Autodesk Inventor part; units mm, degrees
ref_plane "YZ Plane" through (0, 0, 0) normal (1, 0, 0) x (0, 1, 0)
ref_plane "XZ Plane" through (0, 0, 0) normal (0, 1, 0) x (-1, 0, 0)
ref_plane "XY Plane" through (0, 0, 0) normal (0, 0, 1) x (1, 0, 0)
sketch "Sketch1" plane through (0, 0, 0) normal (0, 1, 0) x (-1, 0, 0)
  line L0 (0, 0) -> (3.5, 0)
  line L1 (3.5, 0) -> (3.5, -8)
  line L2 (3.5, -8) -> (0, -8)
  line L3 (0, -8) -> (0, 0)
  line L4 (3.5, 0) -> (11.5, 0)
  line L5 (11.5, 0) -> (11.5, -13.9)
  line L6 (11.5, -13.9) -> (3.5, -13.9)
  line L7 (3.5, -13.9) -> (3.5, 0)
  line L8 (0, 0) -> (-13, 0)
  line L9 (-13, 0) -> (-13, -23)
  line L10 (-13, -23) -> (0, -23)
  line L11 (0, -23) -> (0, 0)
  line L12 (-13, -21) -> (0, -18.118)
  line L13 (-13, 0) -> (11.5, 0)
  line L14 (11.5, 0) -> (11.5, -23)
  line L15 (11.5, -23) -> (-13, -23)
  line L16 (-13, -23) -> (-13, 0)
  line L17 (-13, -23) -> (0, -20.118) construction
  line L18 (11.5, -23) -> (15.5, -23)
  line L19 (15.5, -23) -> (15.5, -18.5)
  line L20 (15.5, -18.5) -> (11.5, -18.5)
  line L21 (11.5, -18.5) -> (11.5, -23)
  line L22 (0, -8) -> (-5, -8)
  line L23 (-5, -8) -> (-5, -12)
  line L24 (-5, -12) -> (0, -12)
  line L25 (0, -12) -> (0, -8)
  line L26 (3.5, -8) -> (-2, -8)
  line L27 (-2, -8) -> (-2, -23)
  line L28 (-2, -23) -> (3.5, -23)
  line L29 (3.5, -23) -> (3.5, -8)
  line L30 (-5, -8) -> (-4, -8)
  line L31 (-4, -8) -> (-4, -9.1)
  line L32 (-4, -9.1) -> (-5, -9.1)
  line L33 (-5, -9.1) -> (-5, -8)
  line L34 (15.5, -20.3397) -> (3.5, -23)
  point P0 (3.5, -8)
  point P1 (0, -8)
  point P2 (0, -23)
  point P3 (11.5, -18.5)
  point P4 (0, -12)
  point P5 (0, -8)
  point P6 (0, -23)
  point P7 (3.5, -8)
  point P8 (-2, -12)
  point P9 (-2, -18.5614)
  point P10 (-4, -8)
  point P11 (-5, -9.1)
  point P12 (3.5, 0)
  point P13 (0, -12)
  dimension "d0" = 3.5
  dimension "d1" = 8
  dimension "d2" = 8
  dimension "d3" = 13.9
  dimension "d6" = 13
  dimension "d7" = 23
  dimension "d9" = 21
  dimension "d35" = 4
  dimension "d36" = 18.5
  dimension "d41" = 4
  dimension "d42" = 12.5
  dimension "d43" = 8.5
  dimension "d44" = 5.5
  dimension "d45" = 1
  dimension "d46" = 1.1
revolve "Revolution1" add sketch "Sketch1" angle 360 about axis through (0, 0, 0) along (-1, 0, 0) contours L2 L7 L29 L15 L11 | L11 L24 L27 L22 | L27 L24 L23 L32 L31 L22 | L12 L27 L10 L9 | L6 L14 L34 L29 | L11 L10 L27 L12 | L20 L19 L34 L14
chamfer "Chamfer2" distance 3.675 distance2 3.5875 1 edges at (-3.5, 0, 8) measured on face at (1.5, 1.2833, -7.8964)
chamfer "Chamfer4" distance 0.5 angle 45 1 edges at (13, 0, 23)
chamfer "Chamfer5" distance 1.5 distance2 3 1 edges at (-11.5, 0, 13.9) measured on face at (-6.1667, 1.1185, -13.8549)
chamfer "Chamfer6" distance 1 angle 45 1 edges at (0, 0, 12)
sketch "Sketch5" plane through (13, 0, 0) normal (1, 0, 0) x (0, 0, -1)
  line L0 (-22, -22) -> (22, -22)
  line L1 (22, -22) -> (22, 22)
  line L2 (22, 22) -> (-22, 22)
  line L3 (-22, 22) -> (-22, -22)
  line L4 (-22, -22) -> (22, 22) construction
  line L5 (22, -22) -> (-22, 22) construction
  circle A0 centre (0, 0) radius 35
  point P0 (0, 0)
  dimension "d53" = 44
  dimension "d54" = 44
  dimension "d55" = 70
equation "\"d53\" = d54"
properties part number "Flywheel" material "Brass, Soft Yellow"
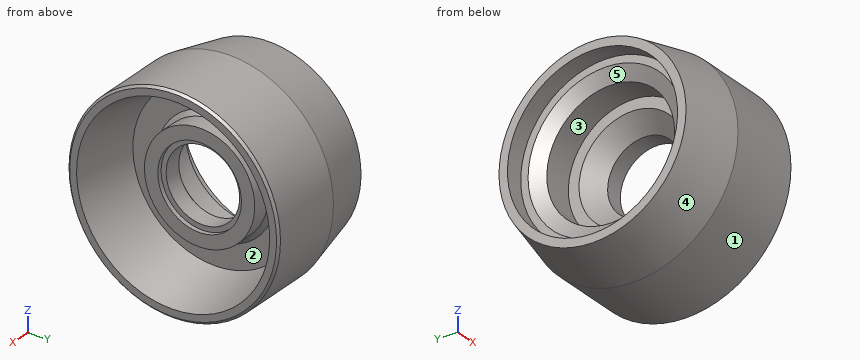
Design review of the part built by this model. Coordinates are the model's own, in mm. Face numbers are marked on the shaded views. A direction names the side the tool comes from. Coordinates: 2 decimals unless noted, no trailing zeros. Order: outer loops, then holes, each group sorted by start corner. A loop starts at its lowest first (then second) coordinate and runs counter-clockwise, first axis right, second up.
1) Wall thickness on line 1 along Z through (x, y) = (1.4, 0); line 2 along Y through (x, z) = (4.55, 0); line 3 along Z through (x, y) = (9.25, -14.5): over which ranges is each line inside the solid? List them lowest first.
2) For the marked faces 1, 2 and 3, list the 3-axis set-ups (+Z, -Z, +X, -X, +Y, -Y) from which the entire face can be reached by the end or side of a thin tool; tool diameter is ignored.
3) Take a section at A-A, the plane x = -6. Give the boundary of the cut face in (y, z).
4) Take a section at B-B, the plane x = 9. Give the boundary of the cut face in (y, z), and give its area (3 significant figures).
5) Clearance check with flat-ended pins moving along their axes: pin 1 (4 mm diameter, centred on x = -10.5, y = -4.5, fed in from +Z); pin 2 (14.5 mm diameter, centred on y = -2.5, z = 1, fed in from +X); pin 3 (4 mm diameter, centred on x = -8, y = -16, fed in from +Z); pin 4 (14.5 mm diameter, centred on y = 0, z = 0, fed in from +X). State where each tip first meets the part, or that it passes through.
6) Mouldability with a two-part tool opening along Y and no side actions: class the marked faces 4 and 5 as +Y half, -Y half, draft (parallel to the pull), parting line (faces both ways), or undercut.
Returned:
1. line 1: z = -23 to -18.43, -12 to -8, 8 to 12, 18.43 to 23
1. line 2: y = -23 to -19.13, -12 to -9.1, 9.1 to 12, 19.13 to 23
1. line 3: z = -17.85 to -14.02, 14.02 to 17.85
2. face 1: +X, -X
2. face 2: +X
2. face 3: -X
3. outline: circle Ø44.89 at (0, 0); hole circle Ø27.8 at (0, 0)
4. outline: circle Ø46 at (0, 0); hole circle Ø40.23 at (0, 0)
4. area: 391 mm2
5. pin 1: stops at z = 21.55
5. pin 2: stops at x = 5
5. pin 3: stops at z = 17.07
5. pin 4: passes through
6. face 4: parting line
6. face 5: undercut
